```python
from build123d import *

# Parameters (mm, degrees)
F1_DEPTH    = 65
F2_DEPTH    = 18
F3_DEPTH    = 65
F4_R        = 5
F5_T1_DEPTH = 18
F7_DEPTH    = 50
F8_R        = 5
F8_R_2      = 2
F9_DEPTH    = 63


# Not quite as in the source:
# - a fillet or chamfer that OpenCascade refuses, or shapes differently, is made with other operations: its cross-section is extruded or revolved along the edge and cut away or added


with BuildPart() as f1:
    # F0 (on Top) → F1 (new body)
    with BuildSketch(Plane.XY):
        with BuildLine():
            ThreePointArc((11, 100), (-4.4397297556, 110.0642336865), (-7.4161453995, 91.8759131335))
            Line((-7.4161453995, 91.8759131335), (-4.039885348, 98.6284332366))
            ThreePointArc((-4.039885348, 98.6284332366), (-1.5492858452, 106.3284184683), (5, 101.5745028853))
            ThreePointArc((5, 101.5745028853), (4.753915583, 100.0252170402), (4.039885348, 98.6284332366))
            Line((4.039885348, 98.6284332366), (7.4161453995, 91.8759131335))
            ThreePointArc((7.4161453995, 91.8759131335), (10.0642336865, 95.5602702444), (11, 100))
        make_face()
        with BuildLine():
            Line((-1.5839824005, 96.8320351991), (-4.9193495505, 90.161300899))
            ThreePointArc((-4.9193495505, 90.161300899), (0, 89), (4.9193495505, 90.161300899))
            Line((4.9193495505, 90.161300899), (1.5839824005, 96.8320351991))
            ThreePointArc((1.5839824005, 96.8320351991), (0, 96.5745028853), (-1.5839824005, 96.8320351991))
        make_face()
        with BuildLine():
            ThreePointArc((-7.4161453995, 91.8759131335), (-6.227044459, 90.9322595259), (-4.9193495505, 90.161300899))
            Line((-4.9193495505, 90.161300899), (-1.5839824005, 96.8320351991))
            ThreePointArc((-1.5839824005, 96.8320351991), (-2.9519033843, 97.5388782237), (-4.039885348, 98.6284332366))
            Line((-4.039885348, 98.6284332366), (-7.4161453995, 91.8759131335))
        make_face()
        with BuildLine():
            Line((1.5839824005, 96.8320351991), (4.9193495505, 90.161300899))
            ThreePointArc((4.9193495505, 90.161300899), (6.227044459, 90.9322595259), (7.4161453995, 91.8759131335))
            Line((7.4161453995, 91.8759131335), (4.039885348, 98.6284332366))
            ThreePointArc((4.039885348, 98.6284332366), (2.9519033843, 97.5388782237), (1.5839824005, 96.8320351991))
        make_face()
        with BuildLine():
            Line((-0.2073593004, 99.5852813993), (-1.5839824005, 96.8320351991))
            ThreePointArc((-1.5839824005, 96.8320351991), (0, 96.5745028853), (1.5839824005, 96.8320351991))
            Line((1.5839824005, 96.8320351991), (0.2073593004, 99.5852813993))
            ThreePointArc((0.2073593004, 99.5852813993), (0, 99.5745028853), (-0.2073593004, 99.5852813993))
        make_face()
        with BuildLine():
            ThreePointArc((-4.039885348, 98.6284332366), (-2.9519033843, 97.5388782237), (-1.5839824005, 96.8320351991))
            Line((-1.5839824005, 96.8320351991), (-0.2073593004, 99.5852813993))
            ThreePointArc((-0.2073593004, 99.5852813993), (-1.7280798318, 100.567656276), (-1.8327895721, 102.3750541855))
            ThreePointArc((-1.8327895721, 102.3750541855), (-2.3164003238, 101.9063812682), (-2.683281573, 101.3416407865))
            Line((-2.683281573, 101.3416407865), (-4.039885348, 98.6284332366))
        make_face()
        with BuildLine():
            ThreePointArc((5, 101.5745028853), (-1.5492858452, 106.3284184683), (-4.039885348, 98.6284332366))
            Line((-4.039885348, 98.6284332366), (-2.683281573, 101.3416407865))
            ThreePointArc((-2.683281573, 101.3416407865), (-2.3164003238, 101.9063812682), (-1.8327895721, 102.3750541855))
            ThreePointArc((-1.8327895721, 102.3750541855), (0, 103.5745028853), (1.8327895721, 102.3750541855))
            ThreePointArc((1.8327895721, 102.3750541855), (2.3164003238, 101.9063812682), (2.683281573, 101.3416407865))
            Line((2.683281573, 101.3416407865), (4.039885348, 98.6284332366))
            ThreePointArc((4.039885348, 98.6284332366), (4.753915583, 100.0252170402), (5, 101.5745028853))
        make_face()
        with BuildLine():
            Line((0.2073593004, 99.5852813993), (1.5839824005, 96.8320351991))
            ThreePointArc((1.5839824005, 96.8320351991), (2.9519033843, 97.5388782237), (4.039885348, 98.6284332366))
            Line((4.039885348, 98.6284332366), (2.683281573, 101.3416407865))
            ThreePointArc((2.683281573, 101.3416407865), (2.3164003238, 101.9063812682), (1.8327895721, 102.3750541855))
            ThreePointArc((1.8327895721, 102.3750541855), (1.9577511517, 101.9834166022), (2, 101.5745028853))
            ThreePointArc((2, 101.5745028853), (1.4857184459, 100.2356075572), (0.2073593004, 99.5852813993))
        make_face()
        with BuildLine():
            ThreePointArc((-1.8327895721, 102.3750541855), (-1.7280798318, 100.567656276), (-0.2073593004, 99.5852813993))
            Line((-0.2073593004, 99.5852813993), (0, 100))
            Line((0, 100), (0.2073593004, 99.5852813993))
            ThreePointArc((0.2073593004, 99.5852813993), (1.4857184459, 100.2356075572), (2, 101.5745028853))
            ThreePointArc((2, 101.5745028853), (1.9577511517, 101.9834166022), (1.8327895721, 102.3750541855))
            ThreePointArc((1.8327895721, 102.3750541855), (0, 103), (-1.8327895721, 102.3750541855))
        make_face()
        with BuildLine():
            Line((0, 100), (-0.2073593004, 99.5852813993))
            ThreePointArc((-0.2073593004, 99.5852813993), (0, 99.5745028853), (0.2073593004, 99.5852813993))
            Line((0.2073593004, 99.5852813993), (0, 100))
        make_face()
        with BuildLine():
            ThreePointArc((1.8327895721, 102.3750541855), (0, 103.5745028853), (-1.8327895721, 102.3750541855))
            ThreePointArc((-1.8327895721, 102.3750541855), (0, 103), (1.8327895721, 102.3750541855))
        make_face()
    extrude(amount=F1_DEPTH)

    # F0 (on Top) → F2 (join)
    with BuildSketch(Plane.XY):
        with BuildLine():
            Line((50, 0), (-50, 0))
            Line((-50, 0), (-4.9193495505, 90.161300899))
            ThreePointArc((-4.9193495505, 90.161300899), (-6.227044459, 90.9322595259), (-7.4161453995, 91.8759131335))
            Line((-7.4161453995, 91.8759131335), (-52.683281573, 1.3416407865))
            ThreePointArc((-52.683281573, 1.3416407865), (-52.5519524251, -1.5771933364), (-50, -3))
            Line((-50, -3), (50, -3))
            ThreePointArc((50, -3), (52.5519524251, -1.5771933364), (52.683281573, 1.3416407865))
            Line((52.683281573, 1.3416407865), (7.4161453995, 91.8759131335))
            ThreePointArc((7.4161453995, 91.8759131335), (6.227044459, 90.9322595259), (4.9193495505, 90.161300899))
            Line((4.9193495505, 90.161300899), (50, 0))
        make_face()
    extrude(amount=F2_DEPTH)

    # F0 (on Top) → F3 (cut)
    with BuildSketch(Plane.XY):
        with BuildLine():
            ThreePointArc((-1.8327895721, 102.3750541855), (-1.7280798318, 100.567656276), (-0.2073593004, 99.5852813993))
            Line((-0.2073593004, 99.5852813993), (0, 100))
            Line((0, 100), (0.2073593004, 99.5852813993))
            ThreePointArc((0.2073593004, 99.5852813993), (1.4857184459, 100.2356075572), (2, 101.5745028853))
            ThreePointArc((2, 101.5745028853), (1.9577511517, 101.9834166022), (1.8327895721, 102.3750541855))
            ThreePointArc((1.8327895721, 102.3750541855), (0, 103), (-1.8327895721, 102.3750541855))
        make_face()
        with BuildLine():
            ThreePointArc((1.8327895721, 102.3750541855), (0, 103.5745028853), (-1.8327895721, 102.3750541855))
            ThreePointArc((-1.8327895721, 102.3750541855), (0, 103), (1.8327895721, 102.3750541855))
        make_face()
        with BuildLine():
            Line((0, 100), (-0.2073593004, 99.5852813993))
            ThreePointArc((-0.2073593004, 99.5852813993), (0, 99.5745028853), (0.2073593004, 99.5852813993))
            Line((0.2073593004, 99.5852813993), (0, 100))
        make_face()
    extrude(amount=F3_DEPTH, mode=Mode.SUBTRACT)

    # F4
    f4_edges = [f1.edges().sort_by_distance(p)[0] for p in [
        (50, 0, 9),
    ]]
    fillet(f4_edges, radius=F4_R)

    # F5: fillet of radius 5 on 5 edges, made by hand

    # F5_s2 → F5_t1 (join)
    with BuildSketch(Plane.XY):
        with BuildLine():
            ThreePointArc((-41.9098300563, 0), (-46.163084098, 2.3713444394), (-46.3819660113, 7.2360679775))
            Line((-46.3819660113, 7.2360679775), (-50, 0))
            Line((-50, 0), (-41.9098300563, 0))
        make_face()
        with BuildLine():
            ThreePointArc((6.7970581872, 86.4058836256), (4.6367553585, 88.6032598618), (1.5983840346, 89.1167482581))
            ThreePointArc((1.5983840346, 89.1167482581), (3.3004522912, 89.5068110341), (4.9193495505, 90.161300899))
            Line((4.9193495505, 90.161300899), (6.7970581872, 86.4058836256))
        make_face()
        with BuildLine():
            ThreePointArc((9.1796312313, 93.9391114136), (8.361173547, 91.4837383605), (8.8800549269, 88.9480940786))
            Line((8.8800549269, 88.9480940786), (7.4161453995, 91.8759131335))
            ThreePointArc((7.4161453995, 91.8759131335), (8.3617669951, 92.8529129906), (9.1796312313, 93.9391114136))
        make_face()
        with BuildLine():
            ThreePointArc((-9.1796312313, 93.9391114136), (-8.361173547, 91.4837383605), (-8.8800549269, 88.9480940786))
            Line((-8.8800549269, 88.9480940786), (-7.4161453995, 91.8759131335))
            ThreePointArc((-7.4161453995, 91.8759131335), (-8.3617669951, 92.8529129906), (-9.1796312313, 93.9391114136))
        make_face()
        with BuildLine():
            ThreePointArc((-1.5983840346, 89.1167482581), (-4.6367553585, 88.6032598618), (-6.7970581872, 86.4058836256))
            Line((-6.7970581872, 86.4058836256), (-4.9193495505, 90.161300899))
            ThreePointArc((-4.9193495505, 90.161300899), (-3.3004522912, 89.5068110341), (-1.5983840346, 89.1167482581))
        make_face()
    extrude(amount=F5_T1_DEPTH)

    # F6 (on face) → F7 (join)
    with BuildSketch(Plane.XY.offset(18)):
        with BuildLine():
            ThreePointArc((41.9098300563, 0), (40.4098300563, -1.5), (41.9098300563, -3))
            Line((41.9098300563, -3), (50, -3))
            ThreePointArc((50, -3), (52.5519524251, -1.5771933364), (52.683281573, 1.3416407865))
            Line((52.683281573, 1.3416407865), (49.0652475842, 8.577708764))
            ThreePointArc((49.0652475842, 8.577708764), (47.0527864045, 9.2485291572), (46.3819660113, 7.2360679775))
            ThreePointArc((46.3819660113, 7.2360679775), (46.163084098, 2.3713444394), (41.9098300563, 0))
        make_face()
        with BuildLine():
            Line((-50, -3), (-41.9098300563, -3))
            ThreePointArc((-41.9098300563, -3), (-40.4098300563, -1.5), (-41.9098300563, 0))
            ThreePointArc((-41.9098300563, 0), (-46.163084098, 2.3713444394), (-46.3819660113, 7.2360679775))
            ThreePointArc((-46.3819660113, 7.2360679775), (-47.0527864045, 9.2485291572), (-49.0652475842, 8.577708764))
            Line((-49.0652475842, 8.577708764), (-52.683281573, 1.3416407865))
            ThreePointArc((-52.683281573, 1.3416407865), (-52.5519524251, -1.5771933364), (-50, -3))
        make_face()
    extrude(amount=F7_DEPTH)

    # F8 (on face) → F9 (cut)
    with BuildSketch(Plane.XY.offset(65)):
        with Locations((0, 101.5745028853)):
            Circle(F8_R)
        with Locations((0, 101.5745028853)):
            Circle(F8_R_2, mode=Mode.SUBTRACT)
    extrude(amount=-F9_DEPTH, mode=Mode.SUBTRACT)


solid = f1.part
```
Check sheet for the modelled part. Datum: model origin and axes. Units: mm. A direction names the side the tool comes from. Give positions to 0.01 mm unless a question says otherwise; leave off trailing zeros. Order: outer loops, then holes, each group sorted by start corner. A loop starts at its lowest first (then second) coordinate and runs counter-clockwise, first axis right, second up. Notation, with made-up numbers: M -37.75,-31.5 L -16.75,-31.5 A10 cw -16.75,-21.5 Z; hole C -36,7.5 d3. An arc over 180 degrees is marked long. Answer in a Markdown table with one row per item. Add a question column.
Q1. Access from +Z, -Z, +X, -X, +Y, -Y to the whole of each face (thin tool, end or side, straight path). Record for faces 1 (the flat face through (23.3, 54.3, 0)), 2 (the flat face through (-27, 46, 9)), 3 (the cylindrical face through (40.41, -1.47, 42.65)).
Q2. Thickness scan on L1, parallel to Y at x = 0, z = 27.5; L2, parallel to X at y = 84, z = 8; L3, parallel to X at y = 101, z = 60. Record the ranges inside material, lowest first.
Q3. Sectioned sample at C-C, the plane y = 44.5. Record the boundary of the cut face in (x, z).
Q4. Sectioned sample at D-D, the plane y = -1.5. Record the boundary of the cut face in (x, z), and give its area (3 significant figures).
Q5. Gauge pin test, flat ends, axial feed: pin 1 Ø6.5 at (x, y) = (-3, 101) entering from +Z; pin 2 Ø4 at (x, z) = (24.5, 15.5) entering from +Y; pin 3 Ø3 at (x, z) = (-8.5, 35) entering from -Y; pin 4 Ø10 at (x, y) = (-23.5, 43) entering from -Z. Record the tip position at first contact, or that the pin passes through.
Q6. Release check for a two-part mould opening along X. For faces 4 (the cylindrical face through (4.68, 88.58, 8.87)), 5 (the cylindrical face through (8.364, 91.52, 8.874)), 6 (the cylindrical face through (-8.364, 91.52, 8.874)) record: released by +X, released by -X, zero draft, split by the parting line, or undercut.
Q7. Sectioned sample at B-B, the plane x = -20.5. Record the boundary of the cut face in (y, z), and give its area (3 significant figures).
Q8. Sectioned sample at A-A, the plane z = 35. Record the boundary of the cut face in (x, y), and give its area (3 significant figures).
Verdict:
| question | item | result |
|---|---|---|
| 1 | face 1 | -Z, +X, -X, +Y, -Y |
| 1 | face 2 | +Z, -Z |
| 1 | face 3 | +Z |
| 2 | L1 | 89 to 96.57, 106.57 to 111 |
| 2 | L2 | -11.35 to -8, 8 to 11.35 |
| 2 | L3 | -10.95 to -4.97, 4.97 to 10.95 |
| 3 | outline | M -31.1,0 L -27.75,0 L -27.75,18 L -31.1,18 Z; M 27.75,0 L 31.1,0 L 31.1,18 L 27.75,18 Z |
| 4 | outline | M -52.6,0 L 52.6,0 L 52.6,68 L 40.41,68 L 40.41,18 L -40.41,18 L -40.41,68 L -52.6,68 Z |
| 4 | area | 3,110 mm² |
| 5 | pin 1 | z = 65 |
| 5 | pin 2 | y = 61.71 |
| 5 | pin 3 | y = 91.51 |
| 5 | pin 4 | z = 0 |
| 6 | face 4 | undercut |
| 6 | face 5 | released by +X |
| 6 | face 6 | released by -X |
| 7 | outline | M -3,0 L 0,0 L 0,18 L -3,18 Z; M 59,0 L 65.71,0 L 65.71,18 L 59,18 Z |
| 7 | area | 175 mm² |
| 8 | outline | M -52.68,1.34 A3 ccw -50,-3 L -41.91,-3 A1.5 ccw -41.91,0 A5 cw -46.38,7.24 A1.5 ccw -49.07,8.58 Z; C 0,100 d22; M 41.91,-3 L 50,-3 A3 ccw 52.68,1.34 L 49.07,8.58 A1.5 ccw 46.38,7.24 A5 cw 41.91,0 A1.5 ccw Z; hole C 0,101.57 d10 |
| 8 | area | 461 mm² |
